Geometry: final body of the model. Coordinates: model frame, mm. A direction names the side the tool comes from. Give positions to 0.01 mm unless a question says otherwise; leave off trailing zeros. Write each loop counter-clockwise with the first axis right and the second up, starting at its lowest first coordinate (ties: lowest second). Pieces come first, ordered by that corner, then holes. Notation, with made-up numbers: (4, 24) -> (29, 24) arc R35 cw to (29, 62) -> close; hole circle Ø9 at (-9, 64.5). An arc over 180 degrees is marked (long way). Answer in a Markdown table with one row per item. Add a question column.
from build123d import *

# Parameters (mm, degrees)
BASE_FLANGE1_DEPTH       = 1
SKETCHED_START           = 21.616422755
SKETCHED_BEND1_OUTLINE_W = 40
SKETCHED_BEND1_OUTLINE_H = 1
SKETCHED_BEND1_DEPTH     = 28.383577245
SKETCHED_START_2         = 20.821902755
SKETCHED_BEND1_2_DEPTH   = 0.00548
SKETCHED_START_3         = 19.821902755
SKETCHED_BEND1_3_DEPTH   = 2
SKETCHED_START_4         = -20
SKETCHED_BEND1_4_DEPTH   = 40
SKETCH7_R                = 3.025
CUT_EXTRUDE1_DEPTH       = 10
F_4_CLEARANCE_HOLE1_D    = 3.2639
F_6_CLEARANCE_HOLE1_D    = 3.7973
F_4_CLEARANCE_HOLE2_D    = 3.2639


with BuildPart() as part:
    # Base-Flange1: sheet metal written as solids
    # Sketch1 → Base-Flange1 (new body)
    with BuildSketch(Plane(origin=(0, 0, 0), x_dir=(1, 0, 0), z_dir=(0, 1, 0))):
        with BuildLine():
            Line((-20, -18), (-20, -45))
            ThreePointArc((-20, -45), (-18.535533906, -48.535533906), (-15, -50))
            Line((-15, -50), (15, -50))
            ThreePointArc((15, -50), (18.535533906, -48.535533906), (20, -45))
            Line((20, -45), (20, -18))
            Line((20, -18), (26, -18))
            ThreePointArc((26, -18), (27.414213562, -17.414213562), (28, -16))
            Line((28, -16), (28, -4))
            ThreePointArc((28, -4), (27.414213562, -2.585786438), (26, -2))
            Line((26, -2), (20, -2))
            Line((20, -2), (20, 35))
            ThreePointArc((20, 35), (15.606601718, 45.606601718), (5, 50))
            Line((5, 50), (-5, 50))
            ThreePointArc((-5, 50), (-15.606601718, 45.606601718), (-20, 35))
            Line((-20, 35), (-20, -2))
            Line((-20, -2), (-26, -2))
            ThreePointArc((-26, -2), (-27.414213562, -2.585786438), (-28, -4))
            Line((-28, -4), (-28, -16))
            ThreePointArc((-28, -16), (-27.414213562, -17.414213562), (-26, -18))
            Line((-26, -18), (-20, -18))
        make_face()
    extrude(amount=-BASE_FLANGE1_DEPTH)

    # Sketched Bend1: read off the stored shape, not the designer's step
    # Sketched Bend1 outline → Sketched Bend1 (cut)
    with BuildSketch(Plane.XY.offset(SKETCHED_START)):
        with Locations((0, -0.5)):
            Rectangle(SKETCHED_BEND1_OUTLINE_W, SKETCHED_BEND1_OUTLINE_H)
    extrude(amount=SKETCHED_BEND1_DEPTH, mode=Mode.SUBTRACT)

    # Sketched Bend1 2 outline → Sketched Bend1 2 (add)
    with BuildSketch(Plane.XY.offset(SKETCHED_START_2)):
        with BuildLine():
            Line((20, 0), (20, 23.821902755))
            ThreePointArc((20, 23.821902755), (18.535533906, 27.357436661), (15, 28.821902755))
            Line((15, 28.821902755), (-15, 28.821902755))
            ThreePointArc((-15, 28.821902755), (-18.535533906, 27.357436661), (-20, 23.821902755))
            Line((-20, 23.821902755), (-20, 0))
            Line((-20, 0), (20, 0))
        make_face()
    extrude(amount=SKETCHED_BEND1_2_DEPTH)

    # Sketched Bend1 3 outline → Sketched Bend1 3 (add)
    with BuildSketch(Plane.XY.offset(SKETCHED_START_3)):
        with BuildLine():
            Line((20, 0), (20, 23.821902755))
            ThreePointArc((20, 23.821902755), (18.535533906, 27.357436661), (15, 28.821902755))
            Line((15, 28.821902755), (-15, 28.821902755))
            ThreePointArc((-15, 28.821902755), (-18.535533906, 27.357436661), (-20, 23.821902755))
            Line((-20, 23.821902755), (-20, 0))
            Line((-20, 0), (20, 0))
        make_face()
    extrude(amount=SKETCHED_BEND1_3_DEPTH)

    # Sketched Bend1 4 outline → Sketched Bend1 4 (cut)
    with BuildSketch(Plane.YZ.offset(SKETCHED_START_4)):
        with BuildLine():
            Line((28.821902755, 19.821902755), (28.821902755, 20.821902755))
            Line((28.821902755, 20.821902755), (1, 20.821902755))
            ThreePointArc((1, 20.821902755), (0.292893219, 20.529009536), (0, 19.821902755))
            Line((0, 19.821902755), (28.821902755, 19.821902755))
        make_face()
        with BuildLine():
            ThreePointArc((-1, 19.821902755), (-0.414213562, 21.236116317), (1, 21.821902755))
            Line((1, 21.821902755), (0, 21.821902755))
            Line((0, 21.821902755), (0, 21.616422755))
            Line((0, 21.616422755), (-1, 21.616422755))
            Line((-1, 21.616422755), (-1, 19.821902755))
        make_face()
    extrude(amount=SKETCHED_BEND1_4_DEPTH, mode=Mode.SUBTRACT)

    # Sketch7 → Cut-Extrude1 (cut)
    with BuildSketch(Plane(origin=(0, 0, 0), x_dir=(1, 0, 0), z_dir=(0, 1, 0))):
        with Locations(Location((0, -6.821902755, 0), (0, 0, 270))):
            Circle(SKETCH7_R)
        with Locations(Location((0, 35.578097245, 0), (0, 0, 270))):
            Circle(SKETCH7_R)
    extrude(amount=-CUT_EXTRUDE1_DEPTH, mode=Mode.SUBTRACT)

    # #4 Clearance Hole1 (through all)
    with Locations(Plane(origin=(0, 0, 0), x_dir=(1, 0, 0), z_dir=(0, 1, 0))):
        with Locations((0, 15.348097245), (-10.21, -6.821902755), (10.21, -6.821902755)):
            Hole(F_4_CLEARANCE_HOLE1_D / 2)

    # #6 Clearance Hole1 (through all)
    with Locations(Plane(origin=(0, 0, 20.821902755), x_dir=(-1, 0, 0), z_dir=(0, 0, -1))):
        with Locations((13, 6.681902755), (-13, 6.681902755), (0, 21.821902755)):
            Hole(F_6_CLEARANCE_HOLE1_D / 2)

    # #4 Clearance Hole2 (through all)
    with Locations(Plane(origin=(0, 0, 0), x_dir=(1, 0, 0), z_dir=(0, 1, 0))):
        with Locations((-24, -6), (-24, -14), (24, -6), (24, -14)):
            Hole(F_4_CLEARANCE_HOLE2_D / 2)


solid = part.part
Q1. Line query: probe 1 along Z at (x, y) = (-24, -0.3); probe 2 along Z at (x, y) = (5.5, 26.5); probe 3 along Y at (x, z) = (18.5, -24). Output: solid intervals per line, ascending. Write a range as from..to.
Q2. Access query for faces 1 (the flat face through (0, 15, 20.822)), 2 (the cylindrical face through (-11.087, -0.507, 5.446)). Directions: +Z, -Z, +X, -X, +Y, -Y. A direction counts if a zero-diameter tool reaches every point of the face in a straight line with its end or side. Return the directions, or none.
Q3. Section A-A on x = 0. Return loops of the section in (y, z).
Q4. Contact query for flat-ended pins moving along their axis: pin 1 Ø2.5 at (x, z) = (-10.21, 6.82) entering from -Y; pin 2 Ø3 at (x, z) = (-15, -18) entering from +Y; pin 3 Ø0.5 at (y, z) = (-0.5, -19) entering from +X; pin 4 Ø1 at (x, y) = (-3, 4) entering from -Z. Output: stop coordinate, or through.
Q5. Section B-B on z = 14. Return loops of the section in (x, y).
Q6. Section D-D on z = 6. Return loops of the section in (x, y).
Q7. Section C-C on x = 24. Return loops of the section in (y, z), and give its area (3 significant figures).
Q8. Pull-direction query (Z, two-part tool) for faces 3 (the flat face through (0, -1, -8)), 4 (the cylindrical face through (-1.2, -0.5, 9.6)), 5 (the flat face through (0, 15, 21.822)); classes: +Z half, -Z half, draft (parallel to the pull), parting line (faces both ways), or undercut.
Checks:
| question | item | result |
|---|---|---|
| 1 | probe 1 | 2..4.37, 7.63..12.37, 15.63..18 |
| 1 | probe 2 | 20.82..21.82 |
| 1 | probe 3 | -1..0 |
| 2 | face 1 | -Z, +X, -X, +Y |
| 2 | face 2 | +Y, -Y |
| 3 | outline | (-1, -50) -> (0, -50) -> (0, -38.6) -> (-1, -38.6) -> close; (-1, -32.55) -> (0, -32.55) -> (0, -16.98) -> (-1, -16.98) -> close; (-1, -13.72) -> (0, -13.72) -> (0, 3.8) -> (-1, 3.8) -> close; (-1, 9.85) -> (0, 9.85) -> (0, 19.82) arc R1 cw to (1, 20.82) -> (19.92, 20.82) -> (19.92, 21.82) -> (1, 21.82) arc R2 ccw to (-1, 19.82) -> close; (23.72, 20.82) -> (28.82, 20.82) -> (28.82, 21.82) -> (23.72, 21.82) -> close |
| 4 | pin 1 | through |
| 4 | pin 2 | y = 0 |
| 4 | pin 3 | x = 20 |
| 4 | pin 4 | z = 20.82 |
| 5 | outline | (-28, -1) -> (-25.63, -1) -> (-25.63, 0) -> (-28, 0) -> close; (-22.37, -1) -> (22.37, -1) -> (22.37, 0) -> (-22.37, 0) -> close; (25.63, -1) -> (28, -1) -> (28, 0) -> (25.63, 0) -> close |
| 6 | outline | (-28, -1) -> (-25.63, -1) -> (-25.63, 0) -> (-28, 0) -> close; (-22.37, -1) -> (-11.62, -1) -> (-11.62, 0) -> (-22.37, 0) -> close; (-8.8, -1) -> (-2.91, -1) -> (-2.91, 0) -> (-8.8, 0) -> close; (2.91, -1) -> (8.8, -1) -> (8.8, 0) -> (2.91, 0) -> close; (11.62, -1) -> (22.37, -1) -> (22.37, 0) -> (11.62, 0) -> close; (25.63, -1) -> (28, -1) -> (28, 0) -> (25.63, 0) -> close |
| 7 | outline | (-1, 2) -> (0, 2) -> (0, 4.37) -> (-1, 4.37) -> close; (-1, 7.63) -> (0, 7.63) -> (0, 12.37) -> (-1, 12.37) -> close; (-1, 15.63) -> (0, 15.63) -> (0, 18) -> (-1, 18) -> close |
| 7 | area | 9.47 mm^2 |
| 8 | face 3 | draft |
| 8 | face 4 | undercut |
| 8 | face 5 | +Z half |
